```python
from build123d import *

# Parameters (mm, degrees)
F0_R      = 5.0038
F0_R_2    = 1.9145814382
F1_DEPTH  = 1.6002
F1_FACE_R = 5.0038
F2_DEPTH  = 0.508
F3_SIZE   = 0.254
F4_R      = 1.9145814382
F4_R_2    = 1.5836825197
F5_DEPTH  = 25.4


with BuildPart() as f1:
    # F0 (on Top) → F1 (new body)
    with BuildSketch(Plane.XY):
        Circle(F0_R)
        Circle(F0_R_2, mode=Mode.SUBTRACT)
        Circle(F0_R_2)
    extrude(amount=F1_DEPTH)

    # F0 (on Top) + F1_face (on face) → F2 (cut)
    with BuildSketch(Plane.XY):
        Circle(F0_R)
        Circle(F0_R_2, mode=Mode.SUBTRACT)
    with BuildSketch(Plane.XY.offset(1.6002)):
        Circle(F1_FACE_R)
    extrude(amount=-F2_DEPTH, mode=Mode.SUBTRACT)

    # F3
    f3_edges = [f1.edges().sort_by_distance(p)[0] for p in [
        (-5.0038, 0, 1.0922),
    ]]
    chamfer(f3_edges, length=F3_SIZE)

    # F4 (on face) → F5 (join)
    with BuildSketch(Plane.XY.offset(1.0922)):
        Circle(F4_R)
        Circle(F4_R_2, mode=Mode.SUBTRACT)
    extrude(amount=-F5_DEPTH)


solid = f1.part
```
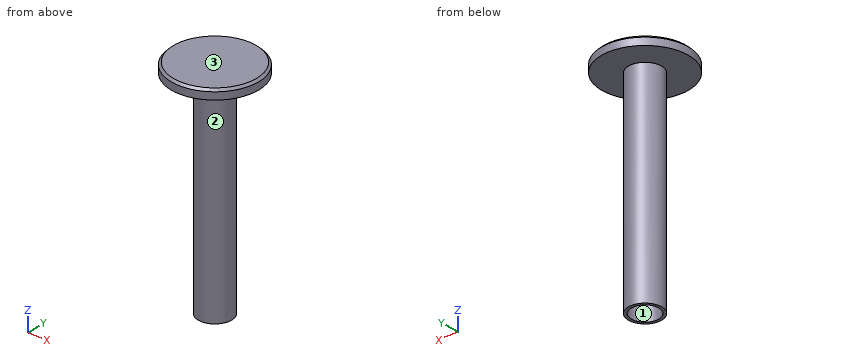
Build history of the part. All positions in model axes, mm. Face numbers are marked on the shaded views. Coordinates: 2 decimals unless noted, no trailing zeros. Order: outer loops, then holes, each group sorted by start corner. A loop starts at its lowest first (then second) coordinate and runs counter-clockwise, first axis right, second up. Notation, with made-up numbers: (45, 89.5) -> (101, 89.5) arc R33 cw to (101, 123.5) -> close; hole circle Ø6 at (61.5, 60.25). An arc over 180 degrees is marked (long way). Answer in a Markdown table with one row per item. Add a question column.
Q1. Band-saw the part on A-A, the plane y = 0. List the corners of the cut face in (x, z).
Q2. Wall check: line 1 along Y through (x, z) = (0, -5); line 2 along Y through (x, z) = (-0.5, -8.75); line 3 along X through (y, z) = (-0.25, -12.75). Give the ranges that are in metal, low to high. Write a range as [from, to].
Q3. Drop flat-ended pins along their axis: pin 1 (5 mm diameter, centred on y = -0.5, z = -9, fed in from -X); pin 2 (5 mm diameter, centred on y = 1.5, z = -18.5, fed in from +X); pin 3 (2.5 mm diameter, centred on x = 0, y = 0, fed in from -Z). Give the stop position or say it passes through.
Q4. Mould opens along X. For the marked faces 1, 2 and 3 say: +X half, -X half, draft (parallel to the pull), parting line (faces both ways), or undercut.
Q5. Band-saw the part on C-C, the plane z = -12.75. List the corners of the cut face in (x, y).
Answers follow:
| question | item | result |
|---|---|---|
| 1 | outline | (-5, 0) -> (-1.91, 0) -> (-1.91, -24.31) -> (-1.58, -24.31) -> (-1.58, 0) -> (1.58, 0) -> (1.58, -24.31) -> (1.91, -24.31) -> (1.91, 0) -> (5, 0) -> (5, 0.84) -> (4.75, 1.09) -> (-4.75, 1.09) -> (-5, 0.84) -> close |
| 2 | line 1 | [-1.91, -1.58], [1.58, 1.91] |
| 2 | line 2 | [-1.85, -1.5], [1.5, 1.85] |
| 2 | line 3 | [-1.9, -1.56], [1.56, 1.9] |
| 3 | pin 1 | x = -1.91 |
| 3 | pin 2 | x = 1.91 |
| 3 | pin 3 | z = 0 |
| 4 | face 1 | undercut |
| 4 | face 2 | parting line |
| 4 | face 3 | draft |
| 5 | outline | circle Ø3.83 at (0, 0); hole circle Ø3.17 at (0, 0) |
